```python
from build123d import *

# Parameters (mm, degrees)
SKETCH_1_W               = 15
SKETCH_1_H               = 8
SKETCH_1_R               = 2.2
SKETCH_1_R_2             = 0.6
EXTRUDE_1_DEPTH          = 3
FILLET_1_R               = 2
SKETCH_2_R               = 1.6
EXTRUDE_2_DEPTH          = 22.5
CUT_EXTRUDE_1_DEPTH      = 43.182233899
CUT_EXTRUDE_1_DEPTH_BACK = 43.182233899
SKETCH_3_W               = 22.164318084
SKETCH_3_H               = 14.5
FILLET_2_R               = 4


with BuildPart() as part:
    # 草图1 → 凸台-拉伸1 (new body)
    with BuildSketch(Plane(origin=(0, 0, 0), x_dir=(1, 0, 0), z_dir=(0, 1, 0))):
        Rectangle(SKETCH_1_W, SKETCH_1_H)
        with Locations(Location((0, 0, 0), (0, 0, 270))):
            Circle(SKETCH_1_R, mode=Mode.SUBTRACT)
        with Locations(Location((-5, 0, 0), (0, 0, 270))):
            Circle(SKETCH_1_R_2, mode=Mode.SUBTRACT)
        with Locations(Location((5, 0, 0), (0, 0, 90))):
            Circle(SKETCH_1_R_2, mode=Mode.SUBTRACT)
    extrude(amount=EXTRUDE_1_DEPTH)

    # 圆角1
    fillet_1_edges = [part.edges().sort_by_distance(p)[0] for p in [
        (7.5, 1.5, 4),
        (7.5, 1.5, -4),
    ]]
    fillet(fillet_1_edges, radius=FILLET_1_R)

    # 草图2 → 凸台-拉伸2 (add)
    with BuildSketch(Plane.XY.offset(4)):
        with BuildLine():
            Line((-7.5, 0), (-7.5, 3))
            Line((-7.5, 3), (-22.5, 3))
            ThreePointArc((-22.5, 3), (-24.864318084, 4.3), (-27.228636167, 3))
            Line((-27.228636167, 3), (-32.5, 3))
            ThreePointArc((-32.5, 3), (-37.664318084, 1.5), (-32.5, 0))
            Line((-32.5, 0), (-27.228636167, 0))
            ThreePointArc((-27.228636167, 0), (-24.864318084, -1.3), (-22.5, 0))
            Line((-22.5, 0), (-7.5, 0))
        make_face()
        with Locations((-24.864318084, 1.5)):
            Circle(SKETCH_2_R, mode=Mode.SUBTRACT)
        with Locations((-34.864318084, 1.5)):
            Circle(SKETCH_2_R, mode=Mode.SUBTRACT)
    extrude(amount=-EXTRUDE_2_DEPTH)

    # 草图3 → 切除-拉伸1 (cut, two sides: drawn at the far end of the back side and taken through both)
    with BuildSketch(Plane(origin=(0, 3, 0), x_dir=(1, 0, 0), z_dir=(0, 1, 0)).offset(-CUT_EXTRUDE_1_DEPTH_BACK)):
        with Locations((-26.582159042, 3.25)):
            Rectangle(SKETCH_3_W, SKETCH_3_H)
    extrude(amount=CUT_EXTRUDE_1_DEPTH + CUT_EXTRUDE_1_DEPTH_BACK, mode=Mode.SUBTRACT)

    # 圆角2
    fillet_2_edges = [part.edges().sort_by_distance(p)[0] for p in [
        (-7.5, 1.5, -18.5),
        (-15.5, 1.5, -10.5),
        (-7.5, 1.5, -4),
        (-15.5, 1.5, 4),
    ]]
    fillet(fillet_2_edges, radius=FILLET_2_R)


solid = part.part
```
Here's how the part is built. I have some questions about the finished solid (model axes, mm). A direction names the side the tool comes from. Coordinates: 2 decimals unless noted, no trailing zeros. Order: outer loops, then holes, each group sorted by start corner. A loop starts at its lowest first (then second) coordinate and runs counter-clockwise, first axis right, second up.
Item 1: If we section it at D-D, the plane z = -3.25: List the corners of the cut face in (x, y) for me.
Response values:
outline: (-15.5, 0) - (7.06, 0) - (7.06, 3) - (-15.5, 3) - close
Item 2: I need wall thicknesses on probe 1 along X at (y, z) = (1.25, -11.75); probe 2 along X at (y, z) = (2.7, -11.75); probe 3 along Y at (x, z) = (-1.5, -2.75). Which ranges of each line are inside material? Lowest first, please.
Response values:
probe 1: x = -37.65 to -36.44, -33.28 to -26.44, -23.28 to -7.5
probe 2: x = -37.39 to -35.92, -33.81 to -25.92, -23.81 to -7.5
probe 3: y = 0 to 3
Item 3: If we section it at C-C, the plane x = 0: List the corners of the cut face in (y, z) for me, then the cut area to 3 significant figures.
Response values:
outline: (0, -4) - (3, -4) - (3, -2.2) - (0, -2.2) - close; (0, 2.2) - (3, 2.2) - (3, 4) - (0, 4) - close
area: 10.8 mm2
Item 4: If we section it at B-B, the plane y = 0.45: List the corners of the cut face in (x, z) for me.
Response values:
outline: (-37.46, -18.5) - (-36.07, -18.5) - (-36.07, -10.5) - (-37.46, -10.5) - close; (-33.66, -18.5) - (-26.07, -18.5) - (-26.07, -10.5) - (-33.66, -10.5) - close; (-23.66, -18.5) - (-11.5, -18.5) arc R4 ccw to (-7.5, -14.5) - (-7.5, -8) arc R4 cw to (-3.5, -4) - (5.5, -4) arc R2 ccw to (7.5, -2) - (7.5, 2) arc R2 ccw to (5.5, 4) - (-11.5, 4) arc R4 ccw to (-15.5, 0) - (-15.5, -6.5) arc R4 cw to (-19.5, -10.5) - (-23.66, -10.5) - close; hole circle Ø1.2 at (-5, 0); hole circle Ø4.4 at (0, 0); hole circle Ø1.2 at (5, 0)
Item 5: Thinking about a two-plate mould opening in Z: for faces 6 (the face through (6.9, 1.52, -3.43)), 7 (the face through (5.586, 1.479, 0.13)), 8 (the face through (-30, 0, -14)), 9 (the face through (-5.586, 1.479, -0.13)), which applies, pulls with the +Z half, pulls with the -Z half, needs draft (parallel to the pull), parting line crosses it, or undercut?
Response values:
face 6: pulls with the -Z half
face 7: undercut
face 8: needs draft
face 9: undercut
Item 6: Which directions (+Z, -Z, +X, -X, +Y, -Y) give clear straight access to the entire face, cutting with the end or side of a thin tool? Please do faces 1 (the face through (-30, 3, -14)), 2 (the face through (-8, 0, -7)), 3 (the face through (-7.5, 1, -11)), 4 (the face through (-11, 3, -5)), 5 (the face through (-29, 1, -10.5)).
Response values:
face 1: +Z, -Z, +Y
face 2: +Z, -Z, +X, -Y
face 3: -Z, +X, +Y, -Y
face 4: +Z, -Z, +X, +Y
face 5: +Z, -X, +Y, -Y
Item 7: I'm going to push flat-ended pins straight in: pin 1 Ø0.7 at (x, z) = (-5, 0) entering from +Y; pin 2 Ø0.9 at (y, z) = (2, -2.5) entering from -X; pin 3 Ø1.6 at (x, z) = (-31, -14.5) entering from -Y; pin 4 Ø0.9 at (x, y) = (-1, 1.5) entering from -Z. Where does each tip first touch, or does it pass through?
Response values:
pin 1: passes through
pin 2: stops at x = -15.5
pin 3: stops at y = 0
pin 4: stops at z = -4
Item 8: If we section it at A-A, the plane x = 5: List the corners of the cut face in (y, z) for me, then the cut area to 3 significant figures.
Response values:
outline: (0, -4) - (3, -4) - (3, -0.6) - (0, -0.6) - close; (0, 0.6) - (3, 0.6) - (3, 4) - (0, 4) - close
area: 20.4 mm2
